For this review, take the finished solid that the model builds, in its own axes (mm). Round coordinates to 2 decimals unless told otherwise and drop trailing zeros. Loops run counter-clockwise (first coordinate to the right, second up) from the corner with the lowest first, then second, coordinate; pieces in that order, holes last. Notation, with made-up numbers: (68.25, -8.5) -> (104.25, -8.5) arc R21 ccw to (104.25, 7.5) -> close; hole circle Ø2 at (-2.75, -19). An arc over 180 degrees is marked (long way). Write each question's results on one line, items separated by ' | '.
Autodesk Inventor part; units mm, degrees
ref_plane "YZ Plane" through (0, 0, 0) normal (1, 0, 0) x (0, 1, 0)
ref_plane "XZ Plane" through (0, 0, 0) normal (0, 1, 0) x (-1, 0, 0)
ref_plane "XY Plane" through (0, 0, 0) normal (0, 0, 1) x (1, 0, 0)
sketch "Sketch1" plane through (0, 0, 0) normal (0, 1, 0) x (-1, 0, 0)
  circle A0 centre (0, 0) radius 4.5
  circle A1 centre (0, 0) radius 4.25
  dimension "d0" = 9
  dimension "d1" = 8.5
sketch "Sketch2" plane through (0, 0, 0) normal (1, 0, 0) x (0, 1, 0)
  line L0 (0, 0) -> (0, -10) construction
  arc A0 (10, -10) -> (0, 0) centre (0, -10) ccw
  dimension "d2" = 10
extrude "Extrusion1" add sketch "Sketch1" against normal blind 10
sketch "Sketch3" plane through (0, 0, 0) normal (0, 1, 0) x (1, 0, 0)
  circle A0 centre (0, 0) radius 4.25
  circle A1 centre (0, 0) radius 4.5
sweep "Sweep1" add profiles "Sketch3" path "Sketch2"
sketch "Sketch4" plane through (0, 10, -10) normal (0, 0, -1) x (-1, 0, 0)
  circle A0 centre (0, 0) radius 4.25
  circle A1 centre (0, 0) radius 4.5
  point P0 (0, -10)
extrude "Extrusion2" add sketch "Sketch4" along normal blind 2
properties part number "Rørende - water block"
1. To check wall thickness, follow probe 1 along X at (y, z) = (-2.5, 0); probe 2 along Y at (x, z) = (0, -10.5). State the ranges of each line that lie inside material, in increasing order.
Values found:
probe 1: x = -4.5 to -4.25, 4.25 to 4.5 | probe 2: y = 5.5 to 5.75, 14.25 to 14.5
2. Draft analysis for pull direction Y (two halves, no side actions). For faces 1 (the face through (0.92, 14.15, -10.99)), 2 (the face through (0.98, 14.39, -10.99)), 3 (the face through (0.59, -4.93, 4.46)), state which applies: released by +Y, released by -Y, zero draft, split by the parting line, or undercut.
Values found:
face 1: undercut | face 2: split by the parting line | face 3: zero draft
3. Consider section B-B (x = 2.5). State the section outline as (y, z) points, plus the area to 3 significant figures.
Values found:
outline: (-10, -3.74) -> (0, -3.74) arc R6.26 cw to (6.26, -10) -> (6.26, -12) -> (6.56, -12) -> (6.56, -10) arc R6.56 ccw to (0, -3.44) -> (-10, -3.44) -> close; (-10, 3.44) -> (0, 3.44) arc R13.44 cw to (13.44, -10) -> (13.44, -12) -> (13.74, -12) -> (13.74, -10) arc R13.74 ccw to (0, 3.74) -> (-10, 3.74) -> close | area: 16.9 mm2
4. Consider section A-A (x = 0). State the section outline as (y, z) points.
Values found:
outline: (-10, -4.5) -> (0, -4.5) arc R5.5 cw to (5.5, -10) -> (5.5, -12) -> (5.75, -12) -> (5.75, -10) arc R5.75 ccw to (0, -4.25) -> (-10, -4.25) -> close; (-10, 4.25) -> (0, 4.25) arc R14.25 cw to (14.25, -10) -> (14.25, -12) -> (14.5, -12) -> (14.5, -10) arc R14.5 ccw to (0, 4.5) -> (-10, 4.5) -> close
5. For pin 1 (3 mm diameter, centred on y = 11.5, z = -3, fed in from +X); pin 2 (1 mm diameter, centred on y = 12, z = -3, fed in from -X); pin 3 (1 mm diameter, centred on x = -0.5, y = 8.5, fed in from +Z), all flat-tipped, find the tip position at first contact; note any pin that passes through.
Values found:
pin 1: stops at x = 4.05 | pin 2: stops at x = -2.96 | pin 3: stops at z = 2.07
